from build123d import *

# Parameters (mm, degrees)
BOSS_EXTRUDE1_DEPTH     = 10
FILLET1_R               = 2
FILLET2_R               = 2
FILLET3_R               = 2
FILLET4_R               = 2
FILLET5_R               = 2
FILLET6_R               = 2
CUT_EXTRUDE3_DEPTH      = 55.419825047
CUT_EXTRUDE3_DEPTH_BACK = 55.419825047
SKETCH4_R               = 1.225
CUT_EXTRUDE4_DEPTH      = 10


with BuildPart() as part:
    # Sketch1 → Boss-Extrude1 (new body)
    with BuildSketch(Plane(origin=(0, 0, 0), x_dir=(1, 0, 0), z_dir=(0, 1, 0))):
        Polygon((-28.953703704, 0), (24.076296296, 0), (24.076296296, -44.98), (8.026296296, -44.98), (8.026296296, -24.78), (-6.973703704, -24.78), (-6.973703704, -44.98), (-28.953703704, -44.98), align=None)
    extrude(amount=BOSS_EXTRUDE1_DEPTH)

    # Fillet1
    fillet1_edges = [part.edges().sort_by_distance(p)[0] for p in [
        (-6.973703704, 5, 24.78),
    ]]
    fillet(fillet1_edges, radius=FILLET1_R)

    # Fillet2
    fillet2_edges = [part.edges().sort_by_distance(p)[0] for p in [
        (8.026296296, 5, 24.78),
    ]]
    fillet(fillet2_edges, radius=FILLET2_R)

    # Fillet3
    fillet3_edges = [part.edges().sort_by_distance(p)[0] for p in [
        (-6.973703704, 5, 44.98),
    ]]
    fillet(fillet3_edges, radius=FILLET3_R)

    # Fillet4
    fillet4_edges = [part.edges().sort_by_distance(p)[0] for p in [
        (8.026296296, 5, 44.98),
    ]]
    fillet(fillet4_edges, radius=FILLET4_R)

    # Fillet5
    fillet5_edges = [part.edges().sort_by_distance(p)[0] for p in [
        (24.076296296, 5, 0),
    ]]
    fillet(fillet5_edges, radius=FILLET5_R)

    # Fillet6
    fillet6_edges = [part.edges().sort_by_distance(p)[0] for p in [
        (24.076296296, 5, 44.98),
    ]]
    fillet(fillet6_edges, radius=FILLET6_R)

    # Sketch4 → Cut-Extrude3 (cut, two sides: drawn at the far end of the back side and taken through both)
    with BuildSketch(Plane(origin=(0, 10, 0), x_dir=(1, 0, 0), z_dir=(0, 1, 0)).offset(-CUT_EXTRUDE3_DEPTH_BACK)):
        with Locations(Location((-6.958703704, -14.825, 0), (0, 0, 270))):
            Circle(SKETCH4_R)
        with Locations(Location((8.231296296, -14.825, 0), (0, 0, 270))):
            Circle(SKETCH4_R)
    extrude(amount=CUT_EXTRUDE3_DEPTH + CUT_EXTRUDE3_DEPTH_BACK, mode=Mode.SUBTRACT)

    # Sketch2 → Cut-Extrude4 (cut)
    with BuildSketch(Plane(origin=(0, 10, 0), x_dir=(1, 0, 0), z_dir=(0, 1, 0))):
        with BuildLine():
            Line((-27.953703704, -6.7), (-27.953703704, -38.28))
            ThreePointArc((-27.953703704, -38.28), (-23.953703704, -42.28), (-19.953703704, -38.28))
            Line((-19.953703704, -38.28), (-19.953703704, -6.7))
            ThreePointArc((-19.953703704, -6.7), (-23.953703704, -2.7), (-27.953703704, -6.7))
        make_face()
    extrude(amount=-CUT_EXTRUDE4_DEPTH, mode=Mode.SUBTRACT)


solid = part.part
The model under review builds one solid part; all positions refer to its coordinate system, in mm. A direction names the side the tool comes from. Round coordinates to 2 decimals unless told otherwise and drop trailing zeros. Loops run counter-clockwise (first coordinate to the right, second up) from the corner with the lowest first, then second, coordinate; pieces in that order, holes last. Notation, with made-up numbers: (-19, 86) -> (29, 86) arc R18 ccw to (29, 121) -> close; hole circle Ø4 at (66, -18). An arc over 180 degrees is marked (long way). Return JSON: item names as keys, results as strings.
(1) For faces 5 (the flat face through (-6.974, 5, 35)), 6 (the flat face through (-28.954, 5, 23)), list the 3-axis set-ups (+Z, -Z, +X, -X, +Y, -Y) from which the entire face can be reached by the end or side of a thin tool; tool diameter is ignored.
Solved:
{"face 5": "+Z, +Y, -Y", "face 6": "+Z, -Z, -X, +Y, -Y"}
(2) For line 1 (X direction, y = 1.5, z = 27.5); line 2 (X direction, y = 4.5, z = 41.5); line 3 (X direction, y = 9.75, z = 10), list the stretches that pass through material, from the lowest coordinate up.
Solved:
{"line 1": "-28.95 to -27.95, -19.95 to -6.97, 8.03 to 24.08", "line 2": "-28.95 to -26.33, -21.58 to -6.97, 8.03 to 24.08", "line 3": "-28.95 to -27.95, -19.95 to 24.08"}
(3) Add section A-A on z = 30.5. Write out the cut boundary in (x, y), plus the area to 3 significant figures.
Solved:
{"outline": "(-28.95, 0) -> (-27.95, 0) -> (-27.95, 10) -> (-28.95, 10) -> close; (-19.95, 0) -> (-6.97, 0) -> (-6.97, 10) -> (-19.95, 10) -> close; (8.03, 0) -> (24.08, 0) -> (24.08, 10) -> (8.03, 10) -> close", "area": "300 mm2"}
(4) Add section D-D on x = 4.5. Write out the cut boundary in (y, z).
Solved:
{"outline": "(0, 0) -> (10, 0) -> (10, 24.78) -> (0, 24.78) -> close"}
(5) For pin 1 (1.5 mm diameter, centred on x = -5, y = 1.5, fed in from +Z); pin 2 (2 mm diameter, centred on x = -1.5, y = 2.5, fed in from +Z), all flat-tipped, find the tip position at first contact; note any pin that passes through.
Solved:
{"pin 1": "z = 24.94", "pin 2": "z = 24.78"}
(6) The part is to be moulded in two halves that separate along Z. For faces 1 (the cylindrical face through (-23.9, 5.1, 2.7)), 2 (the cylindrical face through (-7.544, 5.07, 44.379)), 3 (the cylindrical face through (23.506, 5.07, 0.601)), 4 (the flat face through (-19.954, 5, 23)), say which applies: released by +Z, released by -Z, zero draft, split by the parting line, or undercut.
Solved:
{"face 1": "undercut", "face 2": "released by +Z", "face 3": "released by -Z", "face 4": "undercut"}
(7) Add section C-C on y = 6.5. Write out the cut boundary in (x, z) (3 decimals).
Solved:
{"outline": "(-28.954, 0) -> (22.076, 0) arc R2 ccw to (24.076, 2) -> (24.076, 42.98) arc R2 ccw to (22.076, 44.98) -> (10.026, 44.98) arc R2 ccw to (8.026, 42.98) -> (8.026, 26.78) arc R2 cw to (6.026, 24.78) -> (-4.974, 24.78) arc R2 cw to (-6.974, 26.78) -> (-6.974, 42.98) arc R2 ccw to (-8.974, 44.98) -> (-28.954, 44.98) -> close; hole (-27.954, 6.7) arc R4 ccw to (-19.954, 6.7) -> (-19.954, 38.28) arc R4 ccw to (-27.954, 38.28) -> close; hole circle Ø2.45 at (-6.959, 14.825); hole circle Ø2.45 at (8.231, 14.825)"}
(8) Add section B-B on z = 12.5. Write out the cut boundary in (x, y), plus the area to 3 significant figures.
Solved:
{"outline": "(-28.95, 0) -> (-27.95, 0) -> (-27.95, 10) -> (-28.95, 10) -> close; (-19.95, 0) -> (24.08, 0) -> (24.08, 10) -> (-19.95, 10) -> close", "area": "450 mm2"}
